CAD build for the part. Positions are in the model's coordinates, mm. Face numbers are marked on the shaded views. A direction names the side the tool comes from. Round coordinates to 2 decimals unless told otherwise and drop trailing zeros. Order: outer loops, then holes, each group sorted by start corner. A loop starts at its lowest first (then second) coordinate and runs counter-clockwise, first axis right, second up. Notation, with made-up numbers: M 60,11.25 L 116,11.25 A19 ccw 116,24.25 Z; hole C 28.25,59 d4. An arc over 180 degrees is marked long. Answer as a JSON object with one key per item and string values.
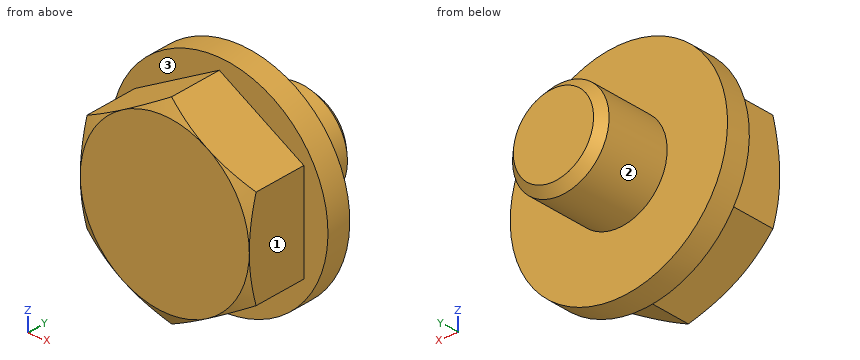
```python
from build123d import *

# Parameters (mm, degrees)
EXTRUDE_1_DEPTH     = 5
SKETCH_3_OUTSIDE_W  = 64.746
SKETCH_3_OUTSIDE_H  = 66.912
SKETCH_3_OUTSIDE_R  = 7
CUT_EXTRUDE_1_DEPTH = 12.80395414
CUT_EXTRUDE_1_DRAFT = -60
SKETCH_4_R          = 9
EXTRUDE_2_DEPTH     = 2
SKETCH_5_R          = 4
EXTRUDE_3_DEPTH     = 6


# Read off the part's stored shape, not the designer's step: M8 机械螺纹 螺柱1
with BuildPart() as part:
    # 草图1 → 凸台-拉伸1 (new body)
    with BuildSketch(Plane(origin=(0, 0, 0), x_dir=(1, 0, 0), z_dir=(0, 1, 0))):
        Polygon((7, -4.041451884), (7, 4.041451884), (0, 8.082903769), (-7, 4.041451884), (-7, -4.041451884), (0, -8.082903769), align=None)
    extrude(amount=EXTRUDE_1_DEPTH)


with BuildPart() as cut_extrude_1_tool:
    # 草图3 outside → 切除-拉伸1 (with draft: the straight prism first)
    with BuildSketch(Plane.XZ):
        Rectangle(SKETCH_3_OUTSIDE_W, SKETCH_3_OUTSIDE_H)
        Circle(SKETCH_3_OUTSIDE_R, mode=Mode.SUBTRACT)
    extrude(amount=-CUT_EXTRUDE_1_DEPTH)
    # 切除-拉伸1: the draft: its side faces are tilted about the plane it starts from
    cut_extrude_1_sides = [cut_extrude_1_tool.faces().sort_by_distance(p)[0] for p in [
        (0, 6.40197707, -33.456),
        (32.373, 6.40197707, 0),
        (0, 6.40197707, 33.456),
        (-32.373, 6.40197707, 0),
        (-7, 6.40197707, 0),
    ]]
    draft(cut_extrude_1_sides, Plane.XZ, CUT_EXTRUDE_1_DRAFT)


with BuildPart() as part_1:
    add(part.part)

    # 切除-拉伸1: cut by cut_extrude_1_tool
    add(cut_extrude_1_tool.part, mode=Mode.SUBTRACT)

    # 草图4 → 凸台-拉伸2 (add)
    with BuildSketch(Plane(origin=(0, 5, 0), x_dir=(1, 0, 0), z_dir=(0, 1, 0))):
        with Locations(Location((0, 0, 0), (0, 0, 270))):
            Circle(SKETCH_4_R)
    extrude(amount=EXTRUDE_2_DEPTH)

    # 草图5 → 凸台-拉伸3 (add)
    with BuildSketch(Plane(origin=(0, 7, 0), x_dir=(1, 0, 0), z_dir=(0, 1, 0))):
        with Locations(Location((0, 0, 0), (0, 0, 270))):
            Circle(SKETCH_5_R)
    extrude(amount=EXTRUDE_3_DEPTH)

    # M8 机械螺纹 螺柱1 outline → M8 机械螺纹 螺柱1 (revolve, cut)
    with BuildSketch(Plane.XY):
        Polygon((4, 13), (3.3235, 13), (4, 12.3235), align=None)
    revolve(axis=Axis((0, 0, 0), (0, 1, 0)), mode=Mode.SUBTRACT)


solid = part_1.part
```
Item 1: Wall check: line 1 along Y through (x, z) = (-7.25, -4.5); line 2 along Y through (x, z) = (0.5, 6.5); line 3 along X through (y, z) = (3.5, 3.5). Give the ranges that are in metal, low to high. Write a range as [from, to].
Worked answers:
{"line 1": "y = [5, 7]", "line 2": "y = [0, 7]", "line 3": "x = [-7, 7]"}
Item 2: Saw through at B-B on y = 5.75. List the corners of the cut face in (x, z), and give its area (3 significant figures).
Worked answers:
{"outline": "C 0,0 d18", "area": "254 mm2"}
Item 3: Drop flat-ended pins along their axis: pin 1 Ø1.5 at (x, y) = (-6, 6) entering from -Z; pin 2 Ø4 at (x, y) = (-5.5, 8) entering from -Z; pin 3 Ø1 at (x, z) = (6.5, -6) entering from -Y. Give the stop position or say it passes through.
Worked answers:
{"pin 1": "stops at z = -7.31", "pin 2": "stops at z = -8.17", "pin 3": "stops at y = 5"}
Item 4: 3-axis set-ups, long thin cutter, end or side, ignore diameter. For the marked faces 1, 2 and 3: which of +Z, -Z, +X, -X, +Y, -Y reach the whole face in a straight line?
Worked answers:
{"face 1": "+Z, -Z, +X, -Y", "face 2": "+Y", "face 3": "-Y"}
Item 5: Saw through at C-C on y = 11. List the corners of the cut face in (x, z), and give its area (3 significant figures).
Worked answers:
{"outline": "C 0,0 d8", "area": "50.3 mm2"}
Item 6: Saw through at A-A on y = 3. List the corners of the cut face in (x, z).
Worked answers:
{"outline": "M -7,-4.04 L 0,-8.08 L 7,-4.04 L 7,4.04 L 0,8.08 L -7,4.04 Z"}
